Verification items for this drawing (mm, ordinates from the low corner). Coordinates: 2 decimals unless noted, no trailing zeros. Order: outer loops, then holes, each group sorted by start corner. A loop starts at its lowest first (then second) coordinate and runs counter-clockwise, first axis right, second up. Notation, with made-up numbers: (41, 38.5) -> (56, 38.5) arc R13 ccw to (56, 51.5) -> close; hole circle Ø4 at (12.5, 9). An arc over 180 degrees is marked (long way). Write each question's results on one line, items separated by ' | '. Start each with the question number.
(1) Cross-section at C-C on x = 179.5. Enter the section's corners in (y, z).
(2) Go/stop test with a flat-tipped pin: pin 1 (3 mm diameter, centred on x = 153.04, z = 7.5, fed in from -Y). Record where the tip stops, or that it passes through.
(3) Thickness scan on probe 1 along Y at (x, z) = (184, 4.25); probe 2 along Z at (x, y) = (175, 0.45). Record the ranges inside material, lowest first. Write a range as [from, to].
(4) Cross-section at A-A on z = 4. Enter the section's corners in (x, y).
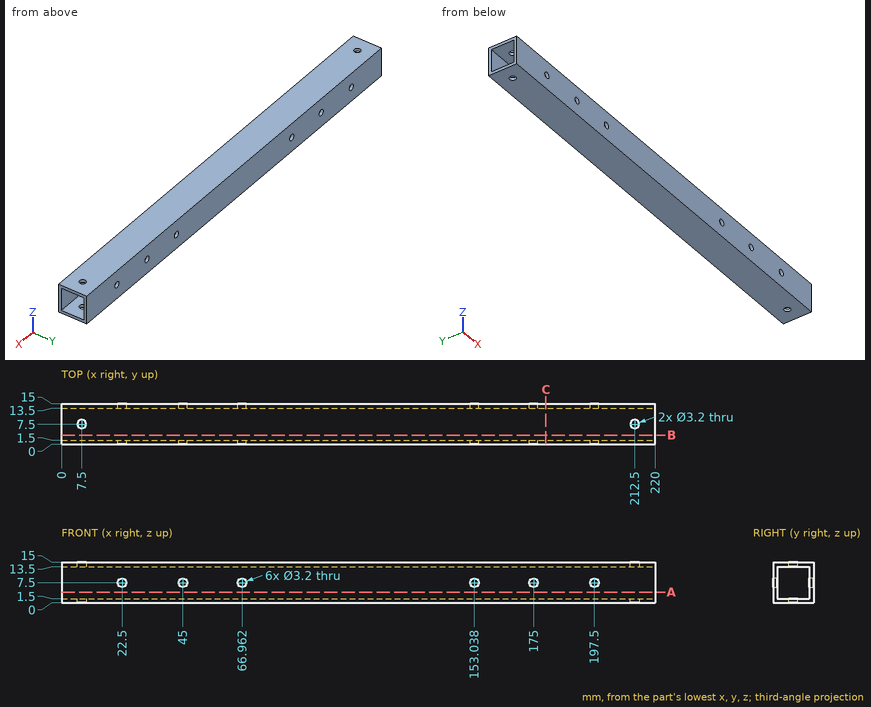
Results are:
1) outline: (0, 0) -> (15, 0) -> (15, 15) -> (0, 15) -> close; hole (1.5, 1.5) -> (13.5, 1.5) -> (13.5, 13.5) -> (1.5, 13.5) -> close
2) pin 1: passes through
3) probe 1: y = [0, 1.5], [13.5, 15] | probe 2: z = [0, 5.9], [9.1, 15]
4) outline: (0, 0) -> (220, 0) -> (220, 1.5) -> (0, 1.5) -> close; (0, 13.5) -> (220, 13.5) -> (220, 15) -> (0, 15) -> close
